```python
from build123d import *

# Parameters (mm, degrees)
F1_DEPTH = 12.7
F2_T     = -2.54
F3_DEPTH = 2.54
F4_R     = 2.54


with BuildPart() as f1:
    # F0 (on Top) → F1 (new body, symmetric)
    with BuildSketch(Plane.XY):
        Polygon((44.9012806053, 44.9012806053), (0, 0), (-44.9012806053, 44.9012806053), (-55.3788052983, 34.4237559124), (-12.7, -8.2550493859), (-38.1, -8.2550493859), (-38.1, -18.4150493859), (-12.7, -18.4150493859), (-12.7, -23.4950493859), (-38.1, -23.4950493859), (-38.1, -33.6550493859), (-12.7, -33.6550493859), (-12.7, -65.7183155417), (12.7, -65.7183155417), (12.7, -33.6550493859), (38.1, -33.6550493859), (38.1, -23.4950493859), (12.7, -23.4950493859), (12.7, -18.4150493859), (38.1, -18.4150493859), (38.1, -8.2550493859), (12.7, -8.2550493859), (55.3788052983, 34.4237559124), align=None)
    extrude(amount=F1_DEPTH, both=True)

    # F2
    f2_openings = [f1.faces().sort_by_distance(p)[0] for p in [
        (0, -9.817912, 12.7),
    ]]
    offset(amount=F2_T, openings=f2_openings, kind=Kind.INTERSECTION)

    # F3 (cut): a face of the model
    f3_faces = [f1.faces().sort_by_distance(p)[0] for p in [
        (0, -9.8179115299, -12.7),
    ]]
    extrude(f3_faces, amount=-F3_DEPTH, mode=Mode.SUBTRACT)

    # F4
    f4_edges = [f1.edges().sort_by_distance(p)[0] for p in [
        (-6.567898, -10.795049, 1.27),
        (6.567898, -10.795049, 1.27),
        (0, -3.592102, 1.27),
    ]]
    fillet(f4_edges, radius=F4_R)


solid = f1.part
```
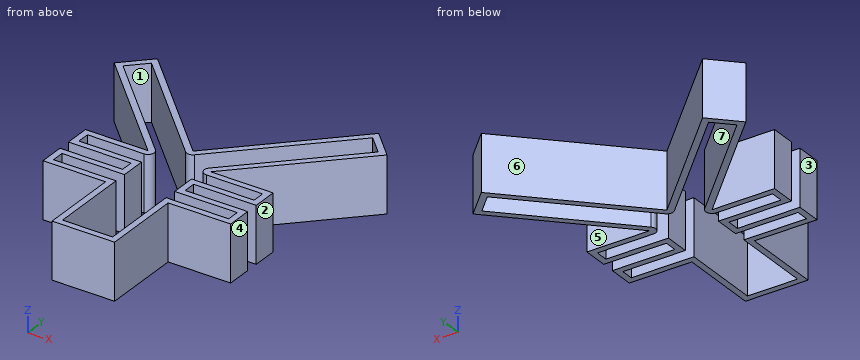
Design review of the part built by this model. Coordinates are the model's own, in mm. Face numbers are marked on the shaded views. A direction names the side the tool comes from. Coordinates: 2 decimals unless noted, no trailing zeros. Order: outer loops, then holes, each group sorted by start corner. A loop starts at its lowest first (then second) coordinate and runs counter-clockwise, first axis right, second up.
1) Take a section at A-A, the plane y = -48. Give the boundary of the cut face in (x, z), and give its area (3 significant figures).
2) For the marked faces 4, 5, 6 and 7, list the 3-axis set-ups (+Z, -Z, +X, -X, +Y, -Y) from which the entire face can be reached by the end or side of a thin tool; tool diameter is ignored.
3) Mouldability with a two-part tool opening along X and no side actions: class the marked faces 1, 2 and 3 as +X half, -X half, draft (parallel to the pull), parting line (faces both ways), or undercut.
4) Clearance check with flat-ended pins moving along their axes: pin 1 (12 mm diameter, centred on x = 33.5, z = -0.5, fed in from +Y); pin 2 (3 mm diameter, centred on y = -13, z = 2, fed in from -X); pin 3 (3 mm diameter, centred on x = 5, z = 4.5, fed in from +Y). State where each tip first meets the part, or that it passes through.
5) Wall thickness on line 1 along Y through (x, z) = (-26.5, 1.25); line 2 along Y through (x, z) = (30.5, -5.25); line 3 along X through (y, z) = (-13, 8.25): over which ranges is each line inside the solid? List them lowest first.
6) Take a section at B-B, the plane x = -47. Give the boundary of the cut face in (y, z).
7) Take a section at D-D, the plane y = 21. Give the boundary of the cut face in (x, z).
8) Take a section at C-C, the plane x = 26. Give the boundary of the cut face in (y, z).
Returned:
1. outline: (-12.7, -10.16) - (-10.16, -10.16) - (-10.16, 12.7) - (-12.7, 12.7) - close; (10.16, -10.16) - (12.7, -10.16) - (12.7, 12.7) - (10.16, 12.7) - close
1. area: 116 mm2
2. face 4: +Z, -Z, +X, -Y
2. face 5: +Z, -Z, +X
2. face 6: +Z, -Z, +Y
2. face 7: +Z, -Z
3. face 1: undercut
3. face 2: +X half
3. face 3: -X half
4. pin 1: stops at y = 39.5
4. pin 2: stops at x = -38.1
4. pin 3: stops at y = 6.5
5. line 1: y = -33.66 to -31.12, -26.04 to -23.5, -18.42 to -15.88, -10.8 to -8.26, 5.54 to 9.14, 22.91 to 26.5
5. line 2: y = -33.66 to -31.12, -26.04 to -23.5, -18.42 to -15.88, -10.8 to -8.26, 9.54 to 13.14, 26.91 to 30.5
5. line 3: x = -38.1 to -35.56, 35.56 to 38.1
6. outline: (26.04, -10.16) - (29.64, -10.16) - (29.64, 12.7) - (26.04, 12.7) - close; (39.21, -10.16) - (42.8, -10.16) - (42.8, 12.7) - (39.21, 12.7) - close
7. outline: (-41.96, -10.16) - (-38.36, -10.16) - (-38.36, 12.7) - (-41.96, 12.7) - close; (-24.59, -10.16) - (-21, -10.16) - (-21, 12.7) - (-24.59, 12.7) - close; (21, -10.16) - (24.59, -10.16) - (24.59, 12.7) - (21, 12.7) - close; (38.36, -10.16) - (41.96, -10.16) - (41.96, 12.7) - (38.36, 12.7) - close
8. outline: (-33.66, -10.16) - (-31.12, -10.16) - (-31.12, 12.7) - (-33.66, 12.7) - close; (-26.04, -10.16) - (-23.5, -10.16) - (-23.5, 12.7) - (-26.04, 12.7) - close; (-18.42, -10.16) - (-15.88, -10.16) - (-15.88, 12.7) - (-18.42, 12.7) - close; (-10.8, -10.16) - (-8.26, -10.16) - (-8.26, 12.7) - (-10.8, 12.7) - close; (5.04, -10.16) - (8.64, -10.16) - (8.64, 12.7) - (5.04, 12.7) - close; (22.41, -10.16) - (26, -10.16) - (26, 12.7) - (22.41, 12.7) - close
